Source: three-view drawing plus pictorial views. Frame: mm from the lowest corner of the part. Coordinates: 2 decimals unless noted, no trailing zeros. Loops run counter-clockwise (first coordinate to the right, second up) from the corner with the lowest first, then second, coordinate; pieces in that order, holes last. Notation, with made-up numbers: M 75,47 L 127,47 A22 cw 127,68 Z; hole C -34.5,-31.5 d10. An arc over 180 degrees is marked long. Write each question's results on one line, items separated by ' | '. Start each with the question number.
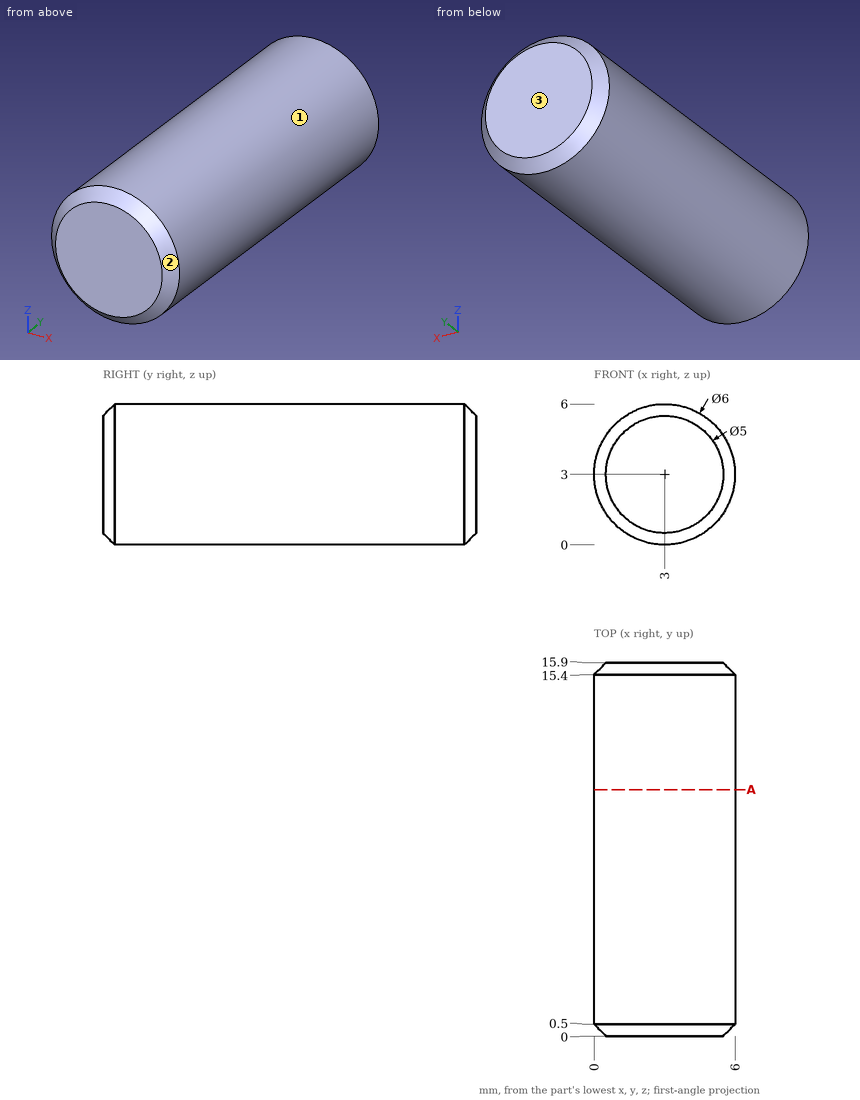
Item 1: Contact query for a flat-ended pin moving along its axis: P1, Ø1, axis at y = 5, z = 4, coming from the -X side. Output: stop coordinate, or through.
Item 2: Ray query, L1, parallel to Z at x = 3.1, y = 6; L2, parallel to X at y = 5.5, z = 4; L3, parallel to X at y = 3.5, z = 4.7. Return the intervals inside material, ascending. Write a range as [from, to].
Item 3: Pull-direction query (Y, two-part tool) for the marked faces 1, 2 and 3; classes: released by +Y, released by -Y, zero draft, split by the parting line, or undercut.
Item 4: Section A-A, the plane y = 10.5. Return loops of the section in (x, z), plus the area to 3 significant figures.
Solutions:
1) P1: stops at x = 0.04
2) L1: z = [0, 6] | L2: x = [0.17, 5.83] | L3: x = [0.53, 5.47]
3) face 1: zero draft | face 2: released by -Y | face 3: released by +Y
4) outline: C 3,3 d6 | area: 28.3 mm²
